Can you work these out from the model? Positions are in its coordinate system, mm. Face numbers are marked on the shaded views. A direction names the side the tool comes from. Coordinates: 2 decimals unless noted, no trailing zeros. Write each loop counter-clockwise with the first axis right and the second up, starting at its lowest first coordinate (ties: lowest second). Pieces come first, ordered by that corner, then holes. Notation, with made-up numbers: M -27.75,60.25 L -21.75,60.25 A26 cw -21.75,82.25 Z; hole C -19,7 d9. An arc over 180 degrees is marked long. Use one line per item in the form item = value. Start each with the question number.
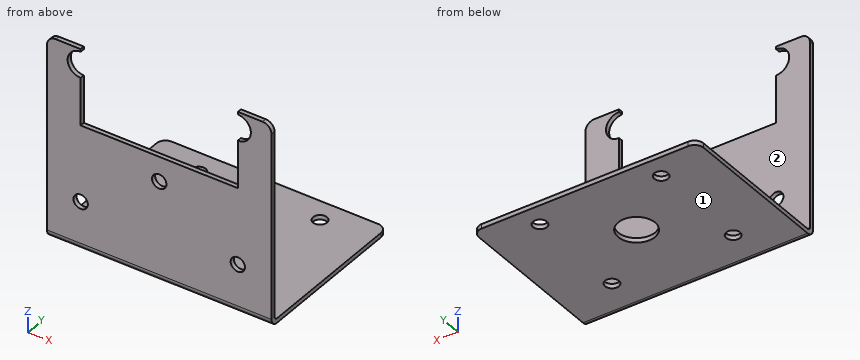
```python
from build123d import *

# Parameters (mm, degrees)
SM_BASE_FLANGE_1_DEPTH           = 1
SM_EDGE_FLANGE_2_STRIP_W         = 5.4732
SM_EDGE_FLANGE_2_STRIP_H         = 1
SM_EDGE_FLANGE_2_STRIP_CUT_DEPTH = 50
SM_EDGE_FLANGE_2_DEPTH           = 50
SKETCH_10_R                      = 1.55
SKETCH_10_R_2                    = 4.1
CUT_EXTRUDE_7_DEPTH              = 10
CUT_EXTRUDE_6_REACH              = 51.267
SKETCH_19_R                      = 2.9
SKETCH_19_R_2                    = 1.6
FILLET_2_R                       = 2


# Sheet-metal steps are written as plain solids
with BuildPart() as part:
    # Sketch 2 → 基体-法兰1 (new body)
    with BuildSketch(Plane(origin=(0, 0, 0), x_dir=(1, 0, 0), z_dir=(0, 1, 0))):
        Polygon((-17.5, -5.5), (17.5, -5.5), (17.5, -22.5), (25, -22.5), (25, 22.5), (-25, 22.5), (-25, -22.5), (-17.5, -22.5), align=None)
    extrude(amount=-SM_BASE_FLANGE_1_DEPTH)

    # 边线-法兰2 strip (across the edge) → 边线-法兰2 strip cut (cut)
    with BuildSketch(Plane(origin=(25, 0, -22.5), x_dir=(0, 0, 1), z_dir=(-1, 0, 0))):
        with Locations((-1, -0.5)):
            Rectangle(SM_EDGE_FLANGE_2_STRIP_W, SM_EDGE_FLANGE_2_STRIP_H)
    extrude(amount=SM_EDGE_FLANGE_2_STRIP_CUT_DEPTH, mode=Mode.SUBTRACT)

    # 边线-法兰2 section (across the edge) → 边线-法兰2 (add)
    with BuildSketch(Plane(origin=(25, 0, -22.5), x_dir=(0, 0, 1), z_dir=(-1, 0, 0))):
        with BuildLine():
            Line((0, 0.7366), (0, 36))
            Line((0, 36), (1, 36))
            Line((1, 36), (1, 0.7366))
            ThreePointArc((1, 0.7366), (1.215745145, 0.215745145), (1.7366, 0))
            Line((1.7366, 0), (1.7366, -1))
            ThreePointArc((1.7366, -1), (0.508638364, -0.491361636), (0, 0.7366))
        make_face()
    extrude(amount=SM_EDGE_FLANGE_2_DEPTH)

    # 草图10 → 切除-拉伸7 (cut)
    with BuildSketch(Plane.XY.offset(-21.5)):
        with Locations((-13.5, 31)):
            Circle(SKETCH_10_R)
        with Locations((13.5, 31)):
            Circle(SKETCH_10_R)
        with Locations((13.5, 8)):
            Circle(SKETCH_10_R)
        with Locations((-13.5, 8)):
            Circle(SKETCH_10_R)
        with Locations((0, 19.5)):
            Circle(SKETCH_10_R_2)
    extrude(amount=-CUT_EXTRUDE_7_DEPTH, mode=Mode.SUBTRACT)

    # 草图19 → 切除-拉伸6 (cut, up to next)
    with BuildSketch(Plane(origin=(0, 0, 0), x_dir=(1, 0, 0), z_dir=(0, 1, 0)), mode=Mode.PRIVATE) as cut_extrude_6_sk1:
        with Locations((-17.5, -19)):
            Circle(SKETCH_19_R)
    cut_extrude_6_tool1 = extrude(cut_extrude_6_sk1.sketch, amount=-CUT_EXTRUDE_6_REACH, mode=Mode.PRIVATE) & part.part
    # 草图19 → 切除-拉伸6 (cut, up to next)
    with BuildSketch(Plane(origin=(0, 0, 0), x_dir=(1, 0, 0), z_dir=(0, 1, 0)), mode=Mode.PRIVATE) as cut_extrude_6_sk2:
        with Locations((17.5, -19)):
            Circle(SKETCH_19_R)
    cut_extrude_6_tool2 = extrude(cut_extrude_6_sk2.sketch, amount=-CUT_EXTRUDE_6_REACH, mode=Mode.PRIVATE) & part.part
    # 草图19 → 切除-拉伸6 (cut, up to next)
    with BuildSketch(Plane(origin=(0, 0, 0), x_dir=(1, 0, 0), z_dir=(0, 1, 0)), mode=Mode.PRIVATE) as cut_extrude_6_sk3:
        with Locations(Location((-17.5, 11.5, 0), (0, 0, 270))):
            Circle(SKETCH_19_R_2)
    cut_extrude_6_tool3 = extrude(cut_extrude_6_sk3.sketch, amount=-CUT_EXTRUDE_6_REACH, mode=Mode.PRIVATE) & part.part
    # 草图19 → 切除-拉伸6 (cut, up to next)
    with BuildSketch(Plane(origin=(0, 0, 0), x_dir=(1, 0, 0), z_dir=(0, 1, 0)), mode=Mode.PRIVATE) as cut_extrude_6_sk4:
        with Locations(Location((17.5, 11.5, 0), (0, 0, 90))):
            Circle(SKETCH_19_R_2)
    cut_extrude_6_tool4 = extrude(cut_extrude_6_sk4.sketch, amount=-CUT_EXTRUDE_6_REACH, mode=Mode.PRIVATE) & part.part
    # 草图19 → 切除-拉伸6 (cut, up to next)
    with BuildSketch(Plane(origin=(0, 0, 0), x_dir=(1, 0, 0), z_dir=(0, 1, 0)), mode=Mode.PRIVATE) as cut_extrude_6_sk5:
        with Locations(Location((0, 0, 0), (0, 0, 270))):
            Circle(SKETCH_19_R_2)
    cut_extrude_6_tool5 = extrude(cut_extrude_6_sk5.sketch, amount=-CUT_EXTRUDE_6_REACH, mode=Mode.PRIVATE) & part.part
    add(cut_extrude_6_tool1.solids().sort_by_distance((-17.5, 0, 19))[0], mode=Mode.SUBTRACT)
    add(cut_extrude_6_tool2.solids().sort_by_distance((17.5, 0, 19))[0], mode=Mode.SUBTRACT)
    add(cut_extrude_6_tool3.solids().sort_by_distance((-17.5, 0, -11.5))[0], mode=Mode.SUBTRACT)
    add(cut_extrude_6_tool4.solids().sort_by_distance((17.5, 0, -11.5))[0], mode=Mode.SUBTRACT)
    add(cut_extrude_6_tool5.solids().sort_by_distance((0, 0, 0))[0], mode=Mode.SUBTRACT)

    # 圆角2
    fillet_2_edges = [part.edges().sort_by_distance(p)[0] for p in [
        (-25, -0.5, 22.5),
        (25, -0.5, 22.5),
        (25, 36, -22),
        (-25, 36, -22),
    ]]
    fillet(fillet_2_edges, radius=FILLET_2_R)


solid = part.part
```
1) Will these pins go through, and if not, where does the flat tip stop? pin 1 Ø0.7 at (y, z) = (-0.5, 22) entering from -X; pin 2 Ø3.5 at (x, z) = (-17.5, -11.5) entering from -Y; pin 3 Ø6 at (x, z) = (-1.5, 7.5) entering from +Y; pin 4 Ø10.5 at (x, y) = (0, 19.5) entering from +Z.
2) Suppose I cut it at C-C on y = 8. Please give me the cut outline in (x, z), and give its area (3 significant figures).
3) Which directions (+Z, -Z, +X, -X, +Y, -Y) give clear straight access to the entire face, cutting with the end or side of a thin tool? Please do the marked faces 1 and 2.
4) Suppose I cut it at D-D on z = 0. Please give me the cut outline in (x, y).
5) Please list where these lines run through material, in increasing order: line 1 (Z direction, x = 7.5, y = 17); line 2 (Y direction, x = 13, z = -22); line 3 (Y direction, x = 15.5, z = -7).
6) Suppose I cut it at A-A on x = 13.5. Please give me the cut outline in (y, z).
7) Suppose I cut it at B-B on z = -11.5. Please give me the cut outline in (x, y).
Computed values:
q1.pin_1 = -24.64
q1.pin_2 = -1
q1.pin_3 = 0
q1.pin_4 = -21.5
q2.outline = M -25,-22.5 L -15.05,-22.5 L -15.05,-21.5 L -25,-21.5 Z; M -11.95,-22.5 L 11.95,-22.5 L 11.95,-21.5 L -11.95,-21.5 Z; M 15.05,-22.5 L 25,-22.5 L 25,-21.5 L 15.05,-21.5 Z
q2.area = 43.8 mm²
q3.face_1 = -Z, +X, -X, +Y, -Y
q3.face_2 = +Z, +X, -X, +Y
q4.outline = M -25,-1 L -1.6,-1 L -1.6,0 L -25,0 Z; M 1.6,-1 L 25,-1 L 25,0 L 1.6,0 Z
q5.line_1 = -22.5 to -21.5
q5.line_2 = -0.48 to 6.53, 9.47 to 29.53, 32.47 to 36
q5.line_3 = -1 to 0
q6.outline = M -1,-20.76 A1.74 ccw 0.74,-22.5 L 6.45,-22.5 L 6.45,-21.5 L 0.74,-21.5 A0.74 cw 0,-20.76 L 0,5.5 L -1,5.5 Z; M 9.55,-22.5 L 29.45,-22.5 L 29.45,-21.5 L 9.55,-21.5 Z; M 32.55,-22.5 L 36,-22.5 L 36,-21.5 L 32.55,-21.5 Z
q7.outline = M -25,-1 L -19.1,-1 L -19.1,0 L -25,0 Z; M -15.9,-1 L 15.9,-1 L 15.9,0 L -15.9,0 Z; M 19.1,-1 L 25,-1 L 25,0 L 19.1,0 Z
